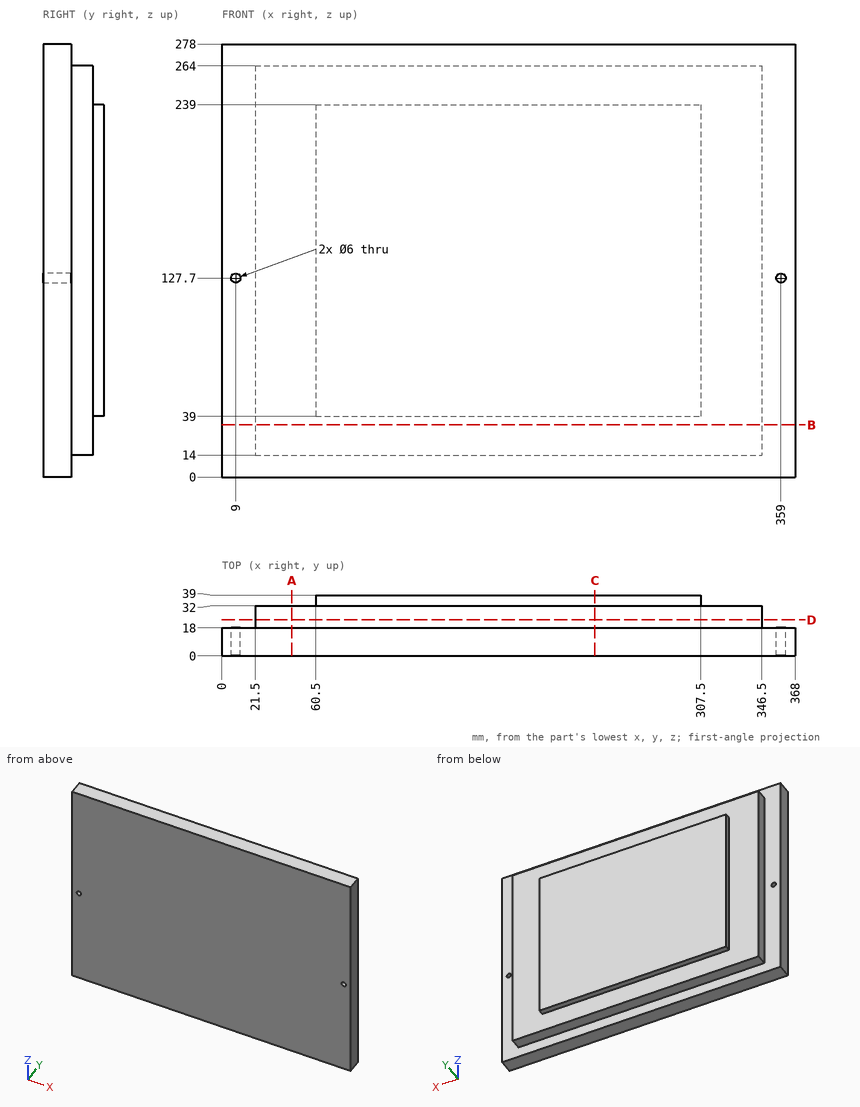
Drawing for the job (mm, zero at the part's lowest x, y, z). Coordinates: 2 decimals unless noted, no trailing zeros. Loops run counter-clockwise (first coordinate to the right, second up) from the corner with the lowest first, then second, coordinate; pieces in that order, holes last. Notation, with made-up numbers: (1.25, 37.25) - (45.25, 37.25) arc R19 cw to (45.25, 53.25) - close; hole circle Ø2 at (25, 35.5). An arc over 180 degrees is marked (long way). Return JSON: item names as keys, results as strings.
1. Drop flat-ended pins along their axis: pin 1 (5 mm diameter, centred on y = 29.5, z = 241, fed in from +X); pin 2 (3.5 mm diameter, centred on x = 9, z = 127.7, fed in from +Y); pin 3 (5.5 mm diameter, centred on y = 36, z = 98, fed in from +X); pin 4 (15.5 mm diameter, centred on x = 188.5, y = 28, fed in from -Z). Give the stop position or say it passes through.
Result:
{"pin 1": "stops at x = 346.5", "pin 2": "passes through", "pin 3": "stops at x = 307.5", "pin 4": "stops at z = 14"}
2. Band-saw the part on A-A (x = 45). Give the cut face in (y, z).
Result:
{"outline": "(0, 0) - (18, 0) - (18, 14) - (32, 14) - (32, 264) - (18, 264) - (18, 278) - (0, 278) - close"}
3. Band-saw the part on C-C (x = 239.5). Give the cut face in (y, z), and give its area (3 significant figures).
Result:
{"outline": "(0, 0) - (18, 0) - (18, 14) - (32, 14) - (32, 39) - (39, 39) - (39, 239) - (32, 239) - (32, 264) - (18, 264) - (18, 278) - (0, 278) - close", "area": "9,900 mm2"}
4. Probe L1, parallel to X at y = 9.25, z = 127.7; L2, parallel to X at y = 7, z = 127; L3, parallel to Z at x = 359, y = 8.5. List the from-to ranges inside material, lowest first. Write a range as from..to.
Result:
{"L1": "x = 0..6, 12..356, 362..368", "L2": "x = 0..6.08, 11.92..356.08, 361.92..368", "L3": "z = 0..124.7, 130.7..278"}
5. Band-saw the part on B-B (z = 33.5). Give the cut face in (x, y).
Result:
{"outline": "(0, 0) - (368, 0) - (368, 18) - (346.5, 18) - (346.5, 32) - (21.5, 32) - (21.5, 18) - (0, 18) - close"}
6. Band-saw the part on D-D (y = 23). Give the cut face in (x, z), and give its area (4 significant figures).
Result:
{"outline": "(21.5, 14) - (346.5, 14) - (346.5, 264) - (21.5, 264) - close", "area": "81,250 mm2"}
